Geometry check sheet. Reference: the model listing, model coordinates, mm. Face numbers are marked on the shaded views. A direction names the side the tool comes from. Round coordinates to 2 decimals unless told otherwise and drop trailing zeros. Order: outer loops, then holes, each group sorted by start corner. A loop starts at its lowest first (then second) coordinate and runs counter-clockwise, first axis right, second up. Notation, with made-up numbers: (28, 82) - (41, 82) arc R23 cw to (41, 113) - close; hole circle Ø7 at (-20, 16.25). An arc over 180 degrees is marked (long way). Answer as CSV lines item,"result". Start each with the question number.
```python
from build123d import *

# Parameters (mm, degrees)
SKETCH1_R           = 30
SKETCH1_R_2         = 15
BOSS_EXTRUDE1_DEPTH = 25
BOSS_EXTRUDE3_DEPTH = 5
SKETCH4_R           = 6
BOSS_EXTRUDE4_DEPTH = 9


with BuildPart() as part:
    # Sketch1 → Boss-Extrude1 (new body, symmetric)
    with BuildSketch(Plane.XY):
        Circle(SKETCH1_R)
        with Locations((0, -1.007153664)):
            Circle(SKETCH1_R_2, mode=Mode.SUBTRACT)
    extrude(amount=BOSS_EXTRUDE1_DEPTH, both=True)

    # Sketch2 → Boss-Extrude3 (add, symmetric)
    with BuildSketch(Plane.XY):
        with BuildLine():
            Line((-122.5, 15), (-122.5, -15))
            Line((-122.5, -15), (-97.5, -15))
            Line((-97.5, -15), (-4.671688756, -29.634023084))
            ThreePointArc((-4.671688756, -29.634023084), (-30, 0), (-4.671688756, 29.634023084))
            Line((-4.671688756, 29.634023084), (-97.5, 15))
            Line((-97.5, 15), (-122.5, 15))
        make_face()
    extrude(amount=BOSS_EXTRUDE3_DEPTH, both=True)

    # Sketch4 → Boss-Extrude4 (add)
    with BuildSketch(Plane(origin=(0, -15, 0), x_dir=(-1, 0, 0), z_dir=(0, -1, 0))):
        with BuildLine():
            Line((122.5, -24), (122.5, -5))
            Line((122.5, -5), (97.5, -5))
            Line((97.5, -5), (97.5, -24))
            ThreePointArc((97.5, -24), (110, -36.5), (122.5, -24))
        make_face()
        with Locations(Location((110, -24, 0), (0, 0, 180))):  # turned: the seam where the file's is
            Circle(SKETCH4_R, mode=Mode.SUBTRACT)
    boss_extrude4 = extrude(amount=-BOSS_EXTRUDE4_DEPTH)

    # Mirror1: Boss-Extrude4 across plane
    add(boss_extrude4.mirror(Plane.ZX))


solid = part.part
```
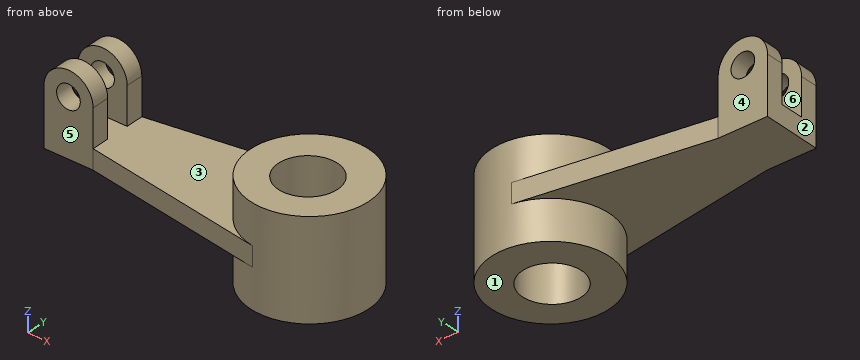
1. Section check D-D on z = 11. Record the boundary of the cut face in (x, y).
2. Draft check along X on the marked faces 1, 2 and 3. Enter one of: released by +X, released by -X, zero draft, split by the parting line, or undercut.
3. Go/stop test with flat-tipped pins: pin 1 Ø4.5 at (y, z) = (8.5, 11) entering from +X; pin 2 Ø12.5 at (x, z) = (-112, 26) entering from -Y; pin 3 Ø5 at (x, y) = (-82.5, -9) entering from +Z; pin 4 Ø7 at (x, z) = (-110, 24) entering from -Y. Record where each tip stops, or that it passes through.
4. Section check A-A on x = -110. Record the boundary of the cut face in (y, z), plus the area to 3 significant figures.
5. Section check B-B on y = -8.5. Record the boundary of the cut face in (x, z), plus the area to 3 significant figures.
6. Access from +Z, -Z, +X, -X, +Y, -Y to the whole of each face (thin tool, end or side, straight path). Record for the marked faces 4, 5 and 6.
7. Section check C-C on x = 0. Record the boundary of the cut face in (y, z), plus the area to 3 significant figures.
8. Thickness scan on probe 1 along Z at (x, y) = (-110, 11); probe 2 along Y at (x, z) = (-111, 32.5); probe 3 along X at (y, z) = (-14, 6). Record the ranges inside material, lowest first.
Numbers:
1,outline,"(-122.5, -15) - (-97.5, -15) - (-97.5, -6) - (-122.5, -6) - close; (-122.5, 6) - (-97.5, 6) - (-97.5, 15) - (-122.5, 15) - close; circle Ø60 at (0, 0); hole circle Ø30 at (0, -1.01)"
2,face 1,"zero draft"
2,face 2,"released by -X"
2,face 3,"undercut"
3,pin 1,"stops at x = 29.34"
3,pin 2,"stops at y = -15"
3,pin 3,"stops at z = 5"
3,pin 4,"passes through"
4,outline,"(-15, -5) - (15, -5) - (15, 18) - (6, 18) - (6, 5) - (-6, 5) - (-6, 18) - (-15, 18) - close; (-15, 30) - (-6, 30) - (-6, 36.5) - (-15, 36.5) - close; (6, 30) - (15, 30) - (15, 36.5) - (6, 36.5) - close"
4,area,"651 mm2"
5,outline,"(-122.5, -5) - (-28.77, -5) - (-28.77, -25) - (-12.99, -25) - (-12.99, 25) - (-28.77, 25) - (-28.77, 5) - (-97.5, 5) - (-97.5, 24) arc R12.5 ccw to (-122.5, 24) - close; (12.99, -25) - (28.77, -25) - (28.77, 25) - (12.99, 25) - close; hole circle Ø12 at (-110, 24)"
5,area,"3,120 mm2"
6,face 4,"+Z, -Z, -X, +Y"
6,face 5,"+Z, -Z, -X, -Y"
6,face 6,"+Z, -X"
7,outline,"(-30, -25) - (-16.01, -25) - (-16.01, 25) - (-30, 25) - close; (13.99, -25) - (30, -25) - (30, 25) - (13.99, 25) - close"
7,area,"1,500 mm2"
8,probe 1,"z = -5 to 18, 30 to 36.5"
8,probe 2,"y = -15 to -6, 6 to 15"
8,probe 3,"x = -122.5 to -97.5, -26.53 to -7.5, 7.5 to 26.53"
